Build history of the part. All positions in model axes, mm. A direction names the side the tool comes from. Coordinates: 2 decimals unless noted, no trailing zeros. Order: outer loops, then holes, each group sorted by start corner. A loop starts at its lowest first (then second) coordinate and runs counter-clockwise, first axis right, second up. Notation, with made-up numbers: (55.25, -5) -> (74.25, -5) arc R16 cw to (74.25, -1) -> close; hole circle Ø5 at (31, -31.75). An arc over 180 degrees is marked (long way). Write each question's results on one line, items separated by ' | '.
from build123d import *

# Parameters (mm, degrees)
SKETCH_1_W          = 18
SKETCH_1_H          = 18
EXTRUDE_1_DEPTH     = 10
SKETCH_2_R          = 1.441488503
SKETCH_2_R_2        = 5.5
CUT_EXTRUDE_1_DEPTH = 10
SKETCH_3_W          = 36
SKETCH_3_H          = 9.968006468
EXTRUDE_2_DEPTH     = 30
SKETCH_4_W          = 10
SKETCH_4_H          = 10
EXTRUDE_3_DEPTH     = 5


with BuildPart() as part:
    # 草图1 → 凸台-拉伸1 (new body)
    with BuildSketch(Plane.XY):
        Rectangle(SKETCH_1_W, SKETCH_1_H)
    extrude(amount=EXTRUDE_1_DEPTH)

    # 草图2 → 切除-拉伸1 (cut)
    with BuildSketch(Plane.XY.offset(10)):
        with Locations((-6, 6)):
            Circle(SKETCH_2_R)
        with Locations((6, 6)):
            Circle(SKETCH_2_R)
        with Locations((6, -6)):
            Circle(SKETCH_2_R)
        with Locations((-6, -6)):
            Circle(SKETCH_2_R)
        Circle(SKETCH_2_R_2)
    extrude(amount=-CUT_EXTRUDE_1_DEPTH, mode=Mode.SUBTRACT)

    # 草图3 → 凸台-拉伸2 (add)
    with BuildSketch(Plane.XZ.offset(9)):
        with Locations((-27, 4.984003234)):
            Rectangle(SKETCH_3_W, SKETCH_3_H)
        with Locations((27, 4.984003234)):
            Rectangle(SKETCH_3_W, SKETCH_3_H)
    extrude(amount=-EXTRUDE_2_DEPTH)

    # 草图4 → 凸台-拉伸3 (add)
    with BuildSketch(Plane.XY.offset(9.968006468)):
        with Locations((40, 16)):
            Rectangle(SKETCH_4_W, SKETCH_4_H)
        with Locations((-40, 16)):
            Rectangle(SKETCH_4_W, SKETCH_4_H)
    extrude(amount=EXTRUDE_3_DEPTH)


solid = part.part
Item 1: Slice it at C-C, the plane x = 0. List the corners of the cut face in (y, z).
Answer:
outline: (-9, 0) -> (-5.5, 0) -> (-5.5, 10) -> (-9, 10) -> close; (5.5, 0) -> (9, 0) -> (9, 10) -> (5.5, 10) -> close
Item 2: Slice it at D-D, the plane z = 2.25. List the corners of the cut face in (x, y), and give its area (3 significant figures).
Answer:
outline: (-45, -9) -> (45, -9) -> (45, 21) -> (9, 21) -> (9, 9) -> (-9, 9) -> (-9, 21) -> (-45, 21) -> close; hole circle Ø2.88 at (-6, -6); hole circle Ø2.88 at (-6, 6); hole circle Ø11 at (0, 0); hole circle Ø2.88 at (6, -6); hole circle Ø2.88 at (6, 6) | area: 2,360 mm^2
Item 3: Tool access for faces 4 (the flat face through (-27, 21, 6)), 5 (the flat face through (35, 16, 12)), 6 (the flat face through (9, 15, 5)), 7 (the flat face through (-1, 6, 0)), 8 (the flat face through (-40, 11, 12)): list every direction of +Z, -Z, +X, -X, +Y, -Y with a clear straight run to the whole face (end or side of a thin tool).
Answer:
face 4: +Z, -Z, +X, -X, +Y | face 5: +Z, +Y, -Y | face 6: +Z, -Z, +Y | face 7: -Z, +X, -X, +Y, -Y | face 8: +Z, +X, -X, -Y
Item 4: Pull direction Y, two halves, no side cores. Call faces 1 (the cylindrical face through (-4.668, 5.448, 5.07)), 2 (the flat face through (27, 6, 9.968)), 3 (the flat face through (40, 11, 12)): released by +Y, released by -Y, zero draft, split by the parting line, or undercut.
Answer:
face 1: undercut | face 2: zero draft | face 3: released by -Y
Item 5: Slice it at B-B, the plane z = 12. List the corners of the cut face in (x, y).
Answer:
outline: (-45, 11) -> (-35, 11) -> (-35, 21) -> (-45, 21) -> close; (35, 11) -> (45, 11) -> (45, 21) -> (35, 21) -> close
Item 6: Drill centre lines: line 1 (Y direction, x = 6, z = 7.5); line 2 (X direction, y = 11.5, z = 12.75); line 3 (X direction, y = 11.5, z = 9.5). Where is each one in solid material? Low to high. Write a range as from..to.
Answer:
line 1: y = -9..-7.44, -4.56..4.56, 7.44..9 | line 2: x = -45..-35, 35..45 | line 3: x = -45..-9, 9..45
Item 7: Pin check, flat tips, straight feed: pin 1 (9 mm diameter, centred on x = -31.5, y = 4.5, fed in from +Z); pin 2 (6 mm diameter, centred on x = -4, z = 7.5, fed in from +Y); pin 3 (1.7 mm diameter, centred on x = 6, y = 6, fed in from -Z). Stop position of each tip, or through.
Answer:
pin 1: stops at z = 9.97 | pin 2: stops at y = 9 | pin 3: passes through
